Design review of the part built by this model. Coordinates are the model's own, in mm. A direction names the side the tool comes from. Give positions to 0.01 mm unless a question says otherwise; leave off trailing zeros. Order: outer loops, then holes, each group sorted by start corner. A loop starts at its lowest first (then second) coordinate and runs counter-clockwise, first axis right, second up. Notation, with made-up numbers: (78.5, 24) -> (93.5, 24) arc R8 cw to (93.5, 37) -> close; hole circle Ø3 at (7, -7). An arc over 180 degrees is marked (long way). One line per item, written item: value.
from build123d import *

# Parameters (mm, degrees)
EXTRUDE_1_DEPTH     = 20
SKETCH_2_R          = 10
CUT_EXTRUDE_1_DEPTH = 20


with BuildPart() as part:
    # 草圖1 → 填料-伸長1 (new body)
    with BuildSketch(Plane.XY):
        with BuildLine():
            Line((-63.548984366, 1.845434638), (-49.394355, 7.7587173))
            ThreePointArc((-49.394355, 7.7587173), (-49.240387651, 8.682408883), (-49.069148505, 9.603054983))
            Line((-49.069148505, 9.603054983), (-60.347687486, 20.00089143))
            ThreePointArc((-60.347687486, 20.00089143), (-60.871436558, 22.155391024), (-59.085335848, 23.469174052))
            Line((-59.085335848, 23.469174052), (-43.761873299, 24.18467377))
            ThreePointArc((-43.761873299, 24.18467377), (-43.301270189, 25), (-42.825478517, 25.806557109))
            Line((-42.825478517, 25.806557109), (-49.867568859, 39.434814809))
            ThreePointArc((-49.867568859, 39.434814809), (-49.622849737, 41.638514912), (-47.49512382, 42.262184708))
            Line((-47.49512382, 42.262184708), (-32.851063821, 37.693601656))
            ThreePointArc((-32.851063821, 37.693601656), (-32.139380484, 38.302222156), (-31.416423783, 38.897407583))
            Line((-31.416423783, 38.897407583), (-33.37268546, 54.112317527))
            ThreePointArc((-33.37268546, 54.112317527), (-32.389014882, 56.099419383), (-30.176298906, 55.957752164))
            Line((-30.176298906, 55.957752164), (-17.977931217, 46.656124884))
            ThreePointArc((-17.977931217, 46.656124884), (-17.101007166, 46.984631039), (-16.218084684, 47.296656639))
            Line((-16.218084684, 47.296656639), (-12.852563667, 62.263076138))
            ThreePointArc((-12.852563667, 62.263076138), (-11.248586821, 63.793905936), (-9.217766989, 62.903988861))
            Line((-9.217766989, 62.903988861), (-0.936394782, 49.991230879))
            ThreePointArc((-0.936394782, 49.991230879), (0, 50), (0.936394782, 49.991230879))
            Line((0.936394782, 49.991230879), (9.217766989, 62.903988861))
            ThreePointArc((9.217766989, 62.903988861), (11.248586821, 63.793905936), (12.852563667, 62.263076138))
            Line((12.852563667, 62.263076138), (16.218084684, 47.296656639))
            ThreePointArc((16.218084684, 47.296656639), (17.101007166, 46.984631039), (17.977931217, 46.656124884))
            Line((17.977931217, 46.656124884), (30.176298906, 55.957752164))
            ThreePointArc((30.176298906, 55.957752164), (32.389014882, 56.099419383), (33.37268546, 54.112317527))
            Line((33.37268546, 54.112317527), (31.416423783, 38.897407583))
            ThreePointArc((31.416423783, 38.897407583), (32.139380484, 38.302222156), (32.851063821, 37.693601656))
            Line((32.851063821, 37.693601656), (47.49512382, 42.262184708))
            ThreePointArc((47.49512382, 42.262184708), (49.622849737, 41.638514912), (49.867568859, 39.434814809))
            Line((49.867568859, 39.434814809), (42.825478517, 25.806557109))
            ThreePointArc((42.825478517, 25.806557109), (43.301270189, 25), (43.761873299, 24.18467377))
            Line((43.761873299, 24.18467377), (59.085335848, 23.469174052))
            ThreePointArc((59.085335848, 23.469174052), (60.871436558, 22.155391024), (60.347687486, 20.00089143))
            Line((60.347687486, 20.00089143), (49.069148505, 9.603054983))
            ThreePointArc((49.069148505, 9.603054983), (49.240387651, 8.682408883), (49.394355, 7.7587173))
            Line((49.394355, 7.7587173), (63.548984366, 1.845434638))
            ThreePointArc((63.548984366, 1.845434638), (64.778029764, 0), (63.548984366, -1.845434638))
            Line((63.548984366, -1.845434638), (49.394355, -7.7587173))
            ThreePointArc((49.394355, -7.7587173), (49.240387651, -8.682408883), (49.069148505, -9.603054983))
            Line((49.069148505, -9.603054983), (60.347687486, -20.00089143))
            ThreePointArc((60.347687486, -20.00089143), (60.871436558, -22.155391024), (59.085335848, -23.469174052))
            Line((59.085335848, -23.469174052), (43.761873299, -24.18467377))
            ThreePointArc((43.761873299, -24.18467377), (43.301270189, -25), (42.825478517, -25.806557109))
            Line((42.825478517, -25.806557109), (49.867568859, -39.434814809))
            ThreePointArc((49.867568859, -39.434814809), (49.622849737, -41.638514912), (47.49512382, -42.262184708))
            Line((47.49512382, -42.262184708), (32.851063821, -37.693601656))
            ThreePointArc((32.851063821, -37.693601656), (32.139380484, -38.302222156), (31.416423783, -38.897407583))
            Line((31.416423783, -38.897407583), (33.37268546, -54.112317527))
            ThreePointArc((33.37268546, -54.112317527), (32.389014882, -56.099419383), (30.176298906, -55.957752164))
            Line((30.176298906, -55.957752164), (17.977931217, -46.656124884))
            ThreePointArc((17.977931217, -46.656124884), (17.101007166, -46.984631039), (16.218084684, -47.296656639))
            Line((16.218084684, -47.296656639), (12.852563667, -62.263076138))
            ThreePointArc((12.852563667, -62.263076138), (11.248586821, -63.793905936), (9.217766989, -62.903988861))
            Line((9.217766989, -62.903988861), (0.936394782, -49.991230879))
            ThreePointArc((0.936394782, -49.991230879), (0, -50), (-0.936394782, -49.991230879))
            Line((-0.936394782, -49.991230879), (-9.217766989, -62.903988861))
            ThreePointArc((-9.217766989, -62.903988861), (-11.248586821, -63.793905936), (-12.852563667, -62.263076138))
            Line((-12.852563667, -62.263076138), (-16.218084684, -47.296656639))
            ThreePointArc((-16.218084684, -47.296656639), (-17.101007166, -46.984631039), (-17.977931217, -46.656124884))
            Line((-17.977931217, -46.656124884), (-30.176298906, -55.957752164))
            ThreePointArc((-30.176298906, -55.957752164), (-32.389014882, -56.099419383), (-33.37268546, -54.112317527))
            Line((-33.37268546, -54.112317527), (-31.416423783, -38.897407583))
            ThreePointArc((-31.416423783, -38.897407583), (-32.139380484, -38.302222156), (-32.851063821, -37.693601656))
            Line((-32.851063821, -37.693601656), (-47.49512382, -42.262184708))
            ThreePointArc((-47.49512382, -42.262184708), (-49.622849737, -41.638514912), (-49.867568859, -39.434814809))
            Line((-49.867568859, -39.434814809), (-42.825478517, -25.806557109))
            ThreePointArc((-42.825478517, -25.806557109), (-43.301270189, -25), (-43.761873299, -24.18467377))
            Line((-43.761873299, -24.18467377), (-59.085335848, -23.469174052))
            ThreePointArc((-59.085335848, -23.469174052), (-60.871436558, -22.155391024), (-60.347687486, -20.00089143))
            Line((-60.347687486, -20.00089143), (-49.069148505, -9.603054983))
            ThreePointArc((-49.069148505, -9.603054983), (-49.240387651, -8.682408883), (-49.394355, -7.7587173))
            Line((-49.394355, -7.7587173), (-63.548984366, -1.845434638))
            ThreePointArc((-63.548984366, -1.845434638), (-64.778029764, 0), (-63.548984366, 1.845434638))
        make_face()
    extrude(amount=EXTRUDE_1_DEPTH)

    # 草圖2 → 除料-伸長1 (cut)
    with BuildSketch(Plane.XY.offset(20)):
        Circle(SKETCH_2_R)
    extrude(amount=-CUT_EXTRUDE_1_DEPTH, mode=Mode.SUBTRACT)


solid = part.part
Item 1: Add section D-D on y = -14. Give the boundary of the cut face in (x, z).
Returned:
outline: (-53.84, 0) -> (53.84, 0) -> (53.84, 20) -> (-53.84, 20) -> close
Item 2: To check wall thickness, follow line 1 along Y through (x, z) = (0, 10); line 2 along Y through (x, z) = (48, 4); line 3 along Y through (x, z) = (58.5, 7). State the ranges of each line that lie inside material, in increasing order. Write a range as from..to.
Returned:
line 1: -50..-10, 10..50
line 2: -42.35..-35.82, -23.99..23.99, 35.82..42.35
line 3: -23.5..-18.3, -3.95..3.95, 18.3..23.5
Item 3: Draft analysis for pull direction Y (two halves, no side actions). For faces 1 (the flat face through (-5.135, 56.538, 9.86)), 2 (the cylindrical face through (60.86, 22.19, 9.86)), 3 (the flat face through (-13, 1, 20)), 4 (the cylindrical face through (-60.86, -22.19, 9.86)), state which applies: pulls with the +Y half, pulls with the -Y half, needs draft (parallel to the pull), parting line crosses it, or undercut.
Returned:
face 1: pulls with the +Y half
face 2: undercut
face 3: needs draft
face 4: undercut
Item 4: Clearance check with flat-ended pins moving along their axes: P1, Ø8, axis at y = -9.5, z = 17.5, coming from the +X side; P2, Ø8, axis at x = -34, z = 3.5, coming from the -Y side; P3, Ø12, axis at y = 14, z = 6.5, coming from the -X side; P4, Ø12, axis at x = 0, y = 0, coming from the -Z side. State where each tip first meets the part, or that it passes through.
Returned:
P1: x = 54.8
P2: y = -56.37
P3: x = -60.35
P4: through
Item 5: Add section A-A on y = 0. Give the boundary of the cut face in (x, z), plus the area to 3 significant figures.
Returned:
outline: (-64.78, 0) -> (-10, 0) -> (-10, 20) -> (-64.78, 20) -> close; (10, 0) -> (64.78, 0) -> (64.78, 20) -> (10, 20) -> close
area: 2,190 mm²
Item 6: Add section B-B on x = 5. Give the boundary of the cut face in (y, z).
Returned:
outline: (-56.33, 0) -> (-8.66, 0) -> (-8.66, 20) -> (-56.33, 20) -> close; (8.66, 0) -> (56.33, 0) -> (56.33, 20) -> (8.66, 20) -> close
Item 7: Add section C-C on x = 36. Give the boundary of the cut face in (y, z).
Returned:
outline: (-38.68, 0) -> (38.68, 0) -> (38.68, 20) -> (-38.68, 20) -> close
Item 8: Machinability: for faces 5 (the flat face through (-32.41, -46.61, 9.86)), 6 (the flat face through (-54.787, -14.875, 9.86)), 7 (the flat face through (54.787, 14.875, 9.86)), 8 (the flat face through (14.512, 54.885, 9.86)), 9 (the flat face through (24.2, -51.4, 9.9)), which of the approach directions +Z, -Z, +X, -X, +Y, -Y give a long, thin tool a straight path to every point of the face, cutting with its end or side? Answer none if there is none.
Returned:
face 5: +Z, -Z
face 6: +Z, -Z, -X
face 7: +Z, -Z, +X
face 8: +Z, -Z, +Y
face 9: +Z, -Z, -Y
